Build history of the part. All positions in model axes, mm. A direction names the side the tool comes from. Give positions to 0.01 mm unless a question says otherwise; leave off trailing zeros. Order: outer loops, then holes, each group sorted by start corner. A loop starts at its lowest first (then second) coordinate and runs counter-clockwise, first axis right, second up. Notation, with made-up numbers: (-31, -31.75) - (24, -31.75) arc R20 cw to (24, -11.75) - close; hole circle Ø5 at (11, 77). An arc over 180 degrees is marked (long way). Answer in a Markdown table with one row per item.
Autodesk Inventor part; units mm, degrees
ref_plane "YZ Plane" through (0, 0, 0) normal (1, 0, 0) x (0, 1, 0)
ref_plane "XZ Plane" through (0, 0, 0) normal (0, 1, 0) x (-1, 0, 0)
ref_plane "XY Plane" through (0, 0, 0) normal (0, 0, 1) x (1, 0, 0)
sketch "Sketch1" plane through (0, 0, 0) normal (0, 1, 0) x (-1, 0, 0)
  circle A0 centre (0, 0) radius 25.5
  circle A1 centre (0, 0) radius 29.5
  dimension "d0" = 51
  dimension "d1" = 59
extrude "Extrusion1" add sketch "Sketch1" along normal blind 5
sketch "Sketch2" plane through (0, 5, 0) normal (0, 1, 0) x (1, 0, 0)
  circle A0 centre (0, -28) radius 1
  point P0 (0, 0)
  dimension "d4" = 2
  dimension "d5" = 28
sketch "Sketch3" plane through (0, 5, 0) normal (0, 1, 0) x (1, 0, 0)
  circle A0 centre (-28, 0) radius 1
  point P0 (0, 0)
  dimension "d6" = 2
  dimension "d7" = 28
sketch "Sketch4" plane through (0, 5, 0) normal (0, 1, 0) x (1, 0, 0)
  circle A0 centre (0, 28) radius 1
  point P0 (0, 0)
  dimension "d8" = 2
  dimension "d9" = 28
sketch "Sketch5" plane through (0, 5, 0) normal (0, 1, 0) x (1, 0, 0)
  circle A0 centre (28, 0) radius 1
  point P0 (0, 0)
  dimension "d10" = 2
  dimension "d11" = 28
hole "Hole1" at (0, 5, 28) direction (0, -1, 0) diameter 2 depth 3 tip angle 118
hole "Hole2" at (-28, 5, 0) direction (0, -1, 0) diameter 2 depth 3 tip angle 118
hole "Hole3" at (0, 5, -28) direction (0, -1, 0) diameter 2 depth 3 tip angle 118
hole "Hole4" at (28, 5, 0) direction (0, -1, 0) diameter 2 depth 3 tip angle 118
thread "Thread1"
thread "Thread2"
thread "Thread3"
thread "Thread4"
properties part number "PMT Cap"
1. Cut at A-A on x = -23. Write the cut outline in (y, z), and give its area (3 significant figures).
Check result:
| item | result |
|---|---|
| outline | (0, -18.47) - (5, -18.47) - (5, -11.01) - (0, -11.01) - close; (0, 11.01) - (5, 11.01) - (5, 18.47) - (0, 18.47) - close |
| area | 74.6 mm² |
2. Which spindle directions (+Z, -Z, +X, -X, +Y, -Y) get a long thin tool onto all of the face, cutting with end or side? Do faces 5 (the face through (13.2, 0, 22)), 6 (the face through (0, 3, -29)). Say none if no direction does.
Check result:
| item | result |
|---|---|
| face 5 | +Z, -Z, +X, -X, -Y |
| face 6 | +Y |
3. Two-plate mould, pull along X, no slides. Class faces 1 (the face through (13.2, 5, 22)), 2 (the face through (-28.14, 2.46, -8.86)), 3 (the face through (28.117, 1.503, -0.128)), 4 (the face through (0.01, 1.5, 27.83)): +X half, -X half, draft (parallel to the pull), parting line (faces both ways), or undercut.
Check result:
| item | result |
|---|---|
| face 1 | draft |
| face 2 | parting line |
| face 3 | undercut |
| face 4 | undercut |
4. Cut at B-B on z = -15. Write the cut outline in (x, y).
Check result:
| item | result |
|---|---|
| outline | (-25.4, 0) - (-20.62, 0) - (-20.62, 5) - (-25.4, 5) - close; (20.62, 0) - (25.4, 0) - (25.4, 5) - (20.62, 5) - close |
5. Cut at C-C on y = 4. Write the cut outline in (x, z).
Check result:
| item | result |
|---|---|
| outline | circle Ø59 at (0, 0); hole circle Ø2 at (-28, 0); hole circle Ø51 at (0, 0); hole circle Ø2 at (0, -28); hole circle Ø2 at (0, 28); hole circle Ø2 at (28, 0) |
6. Drop flat-ended pins along their axis: P1, Ø1, axis at y = 2.5, z = 6, coming from the -X side; P2, Ø1.5, axis at y = 2, z = -16.5, coming from the +X side. Give the stop position or say it passes through.
Check result:
| item | result |
|---|---|
| P1 | stops at x = -28.98 |
| P2 | stops at x = 24.94 |
7. Probe line 1 (Z direction, x = 0, y = 3.35); line 2 (X direction, y = 3.95, z = 23); line 3 (X direction, y = 0.65, z = 2). List the from-to ranges inside material, lowest first.
Check result:
| item | result |
|---|---|
| line 1 | z = -29.5 to -29, -27 to -25.5, 25.5 to 27, 29 to 29.5 |
| line 2 | x = -18.47 to -11.01, 11.01 to 18.47 |
| line 3 | x = -29.43 to -25.42, 25.42 to 29.43 |
